Work out the finished part from the listing and answer in its coordinate system (mm). A direction names the side the tool comes from. Give positions to 0.01 mm unless a question says otherwise; leave off trailing zeros. Write each loop counter-clockwise with the first axis right and the second up, starting at its lowest first coordinate (ties: lowest second). Pieces come first, ordered by that corner, then holes. Notation, with made-up numbers: (-6.5, 6) -> (42.5, 6) arc R8 ccw to (42.5, 12) -> close; hole circle Ø7 at (77, -8.5). An arc over 180 degrees is marked (long way). Write item = value, one per line. Start each with the question number.
from build123d import *

# Parameters (mm, degrees)
BOSS_EXTRUDE1_DEPTH = 15
SKETCH5_R           = 12.5
CUT_EXTRUDE1_DEPTH  = 59
CUT_EXTRUDE3_DEPTH  = 110
SKETCH10_R          = 12.5
CUT_EXTRUDE4_DEPTH  = 94


with BuildPart() as part:
    # Sketch2 → Boss-Extrude1 (new body, symmetric)
    with BuildSketch(Plane.XY):
        with BuildLine():
            Line((-50, -150), (-50, 150))
            ThreePointArc((-50, 150), (0, 200), (50, 150))
            Line((50, 150), (50, -150))
            ThreePointArc((50, -150), (0, -200), (-50, -150))
        make_face()
    extrude(amount=BOSS_EXTRUDE1_DEPTH, both=True)

    # Sketch5 → Cut-Extrude1 (cut)
    with BuildSketch(Plane(origin=(0, 150, 0), x_dir=(1, 0, 0), z_dir=(0, 1, 0))):
        Circle(SKETCH5_R)
    extrude(amount=CUT_EXTRUDE1_DEPTH, mode=Mode.SUBTRACT)

    # Sketch7 → Cut-Extrude3 (cut)
    with BuildSketch(Plane(origin=(50, 0, 0), x_dir=(0, 0, -1), z_dir=(1, 0, 0))):
        Polygon((-15, 130), (0, 121.339745962), (0, -121.339745962), (-15, -130), align=None)
    extrude(amount=-CUT_EXTRUDE3_DEPTH, mode=Mode.SUBTRACT)

    # Sketch10 → Cut-Extrude4 (cut)
    with BuildSketch(Plane(origin=(0, -150, 0), x_dir=(1, 0, 0), z_dir=(0, 1, 0))):
        Circle(SKETCH10_R)
    extrude(amount=-CUT_EXTRUDE4_DEPTH, mode=Mode.SUBTRACT)


solid = part.part
(1) Determine the mould class of faces 1 (the cylindrical face through (11.923, -174.662, -3.755)), 2 (the cylindrical face through (1.099, -199.988, -13.123)), 3 (the flat face through (1, 2, 0)), 4 (the flat face through (0.7, 125.73, 7.605)) for opening direction Y: pulls with the +Y half, pulls with the -Y half, needs draft (parallel to the pull), parting line crosses it, or undercut.
(2) A cutting plane is placed at A-A, the plane z = 6. Write down the section's boundary in (x, y), then the cut area to 3 significant figures.
(3) A cutting plane is placed at B-B, the plane x = 0. Write down the section's boundary in (y, z), then the cut area to 3 significant figures.
(4) A cutting plane is placed at C-C, the plane y = 30. Write down the section's boundary in (x, z), then the cut area to 3 significant figures.
(5) For faces 5 (the flat face through (0, -150, 0)), 6 (the flat face through (50, 2, -6)), 7 (the cylindrical face through (-1.099, 199.988, -13.123)), 8 (the flat face through (0.7, -125.61, 7.4)), 9 (the cylindrical face through (11.923, 174.662, -3.755)), determine the directions among +Z, -Z, +X, -X, +Y, -Y from which every point of the face is accessible in a straight line to the end or side of a thin tool.
(6) Each of these flat-tipped pins is pushed along its axis until it touches: pin 1 (10 mm diameter, centred on x = -37.5, z = 11.5, fed in from -Y); pin 2 (10 mm diameter, centred on x = -15, z = -11.5, fed in from -Y); pin 3 (5 mm diameter, centred on x = -26, z = -3.5, fed in from -Y). Where does it stop, or does it pass through?
(7) A cutting plane is placed at D-D, the plane x = -28.5. Write down the section's boundary in (y, z).
(8) Find the intervals of material crossed by line 1 along Z through (x, y) = (0, 182); line 2 along Z through (x, y) = (25, -94); line 3 along Y through (x, z) = (7.5, -3), in increasing order.
Results list:
q1.face_1 = needs draft
q1.face_2 = pulls with the -Y half
q1.face_3 = undercut
q1.face_4 = undercut
q2.outline = (-50, -150) arc R50 ccw to (-10.97, -198.78) -> (-10.97, -150) -> (10.97, -150) -> (10.97, -198.78) arc R50 ccw to (50, -150) -> (50, -124.8) -> (-50, -124.8) -> close; (-50, 124.8) -> (50, 124.8) -> (50, 150) arc R50 ccw to (10.97, 198.78) -> (10.97, 150) -> (-10.97, 150) -> (-10.97, 198.78) arc R50 ccw to (-50, 150) -> close
q2.area = 10,700 mm²
q3.outline = (-200, -15) -> (200, -15) -> (200, -12.5) -> (150, -12.5) -> (150, 12.5) -> (200, 12.5) -> (200, 15) -> (130, 15) -> (121.34, 0) -> (-121.34, 0) -> (-130, 15) -> (-200, 15) -> (-200, 12.5) -> (-150, 12.5) -> (-150, -12.5) -> (-200, -12.5) -> close
q3.area = 5,730 mm²
q4.outline = (-50, -15) -> (50, -15) -> (50, 0) -> (-50, 0) -> close
q4.area = 1,500 mm²
q5.face_5 = -Y
q5.face_6 = +Z, -Z, +X, +Y, -Y
q5.face_7 = +Z, -Z, +Y
q5.face_8 = +Z, +X, -X
q5.face_9 = +Y
q6.pin_1 = -188
q6.pin_2 = -198.99
q6.pin_3 = -194.13
q7.outline = (-191.08, -15) -> (191.08, -15) -> (191.08, 15) -> (130, 15) -> (121.34, 0) -> (-121.34, 0) -> (-130, 15) -> (-191.08, 15) -> close
q8.line_1 = -15 to -12.5, 12.5 to 15
q8.line_2 = -15 to 0
q8.line_3 = -150 to 150
